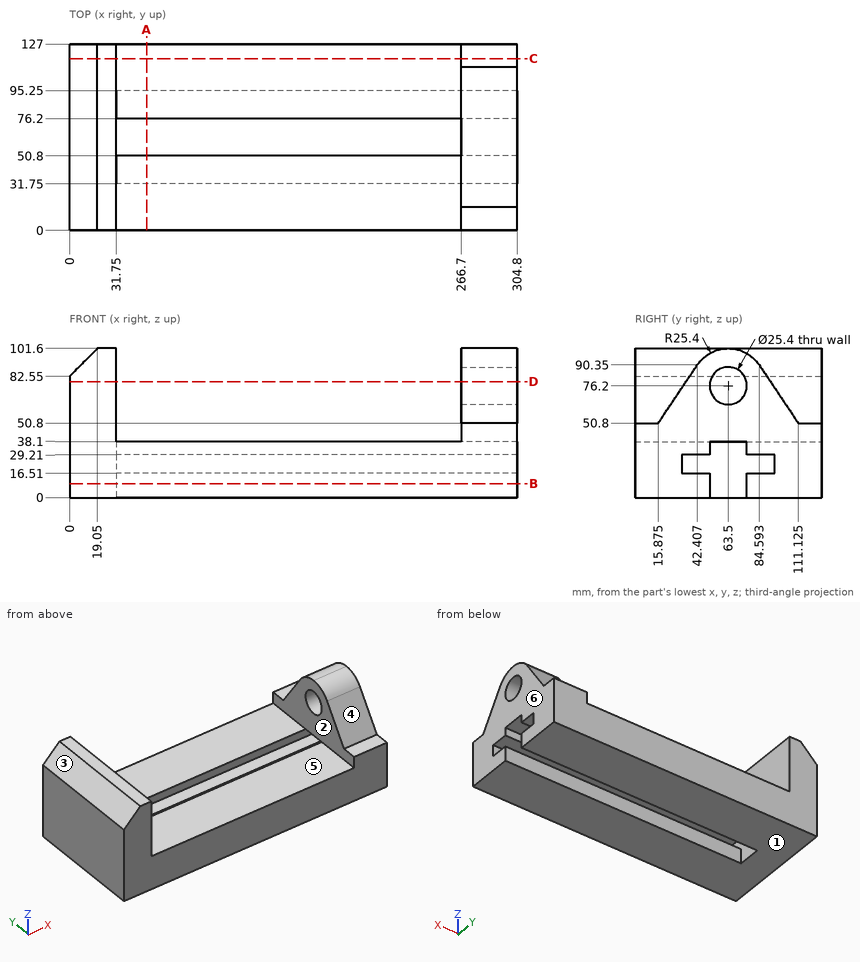
Part print with two shaded views. Sizes in mm from the minimum x, y, z corner. A direction names the side the tool comes from. Coordinates: 2 decimals unless noted, no trailing zeros. Write each loop counter-clockwise with the first axis right and the second up, starting at its lowest first coordinate (ties: lowest second). Pieces come first, ordered by that corner, then holes. Notation, with made-up numbers: (74, 54) - (130, 54) arc R6 ccw to (130, 65) - close; hole circle Ø9 at (53.5, 29). An arc over 180 degrees is marked (long way). One line per item, written item: value. Start each with the question number.
1. Slice it at D-D (z = 79). Write the cut outline in (x, y).
2. Slice it at A-A (x = 52.5). Write the cut outline in (y, z).
3. Tool access for the marked faces 4, 5 and 6: list every direction of +Z, -Z, +X, -X, +Y, -Y with a clear straight run to the whole face (end or side of a thin tool).
4. Slice it at C-C (y = 117). Write the cut outline in (x, z).
5. Mould opens along X. For the marked faces 1, 2 and 3 say: released by +X, released by -X, zero draft, split by the parting line, or undercut.
6. Probe line 1 (Y direction, x = 43, z = 12); line 2 (Z direction, x = 296, y = 63) (1 decimal); line 3 (X direction, y = 55, z = 57). List the from-to ranges inside material, lowest first. Write a range as from..to.
7. Slice it at B-B (z = 9.5). Write the cut outline in (x, y), plus the area to 3 significant figures.
8. Flat gauge pins, fed straight in: pin 1 (2 mm diameter, centred on x = 215, y = 23.5, fed in from +Z); pin 2 (8 mm diameter, centred on x = 279, y = 7.5, fed in from +Z). Where does each tip first touch, or does it go through?
Answers below:
1. outline: (0, 0) - (31.75, 0) - (31.75, 127) - (0, 127) - close; (266.7, 34.79) - (304.8, 34.79) - (304.8, 51.11) - (266.7, 51.11) - close; (266.7, 75.89) - (304.8, 75.89) - (304.8, 92.21) - (266.7, 92.21) - close
2. outline: (0, 0) - (50.8, 0) - (50.8, 16.51) - (31.75, 16.51) - (31.75, 29.21) - (50.8, 29.21) - (50.8, 38.1) - (0, 38.1) - close; (76.2, 0) - (127, 0) - (127, 38.1) - (76.2, 38.1) - (76.2, 29.21) - (95.25, 29.21) - (95.25, 16.51) - (76.2, 16.51) - close
3. face 4: +Z, +X, -Y
3. face 5: +Z, +Y, -Y
3. face 6: +Z, -Z, +X, +Y, -Y
4. outline: (0, 0) - (304.8, 0) - (304.8, 50.8) - (266.7, 50.8) - (266.7, 38.1) - (31.75, 38.1) - (31.75, 101.6) - (19.05, 101.6) - (0, 82.55) - close
5. face 1: zero draft
5. face 2: undercut
5. face 3: released by -X
6. line 1: y = 0..50.8, 76.2..127
6. line 2: z = 38.1..63.5, 88.9..101.6
6. line 3: x = 0..31.75, 266.7..304.8
7. outline: (0, 0) - (304.8, 0) - (304.8, 50.8) - (31.75, 50.8) - (31.75, 76.2) - (304.8, 76.2) - (304.8, 127) - (0, 127) - close
7. area: 31,800 mm^2
8. pin 1: stops at z = 38.1
8. pin 2: stops at z = 50.8
